The listing builds one solid part. Answer for the finished solid, in the listing's coordinates (mm). A direction names the side the tool comes from. Coordinates: 2 decimals unless noted, no trailing zeros. Loops run counter-clockwise (first coordinate to the right, second up) from the corner with the lowest first, then second, coordinate; pieces in that order, holes last. Notation, with made-up numbers: (48, 79) - (59, 79) arc R18 ccw to (59, 103) - close; hole circle Ø10 at (-12.75, -10.5). An arc over 180 degrees is marked (long way). One line per question, with ' | ' between items.
from build123d import *

# Parameters (mm, degrees)
BOSS_EXTRUDE1_DEPTH      = 6.8
BOSS_EXTRUDE1_DEPTH_BACK = 6.8
CUT_EXTRUDE1_REACH       = 45.967
SKETCH2_R                = 1.1303
SKETCH2_R_2              = 1.7272


with BuildPart() as part:
    # Sketch1 → Boss-Extrude1 (new, two sides: drawn at the far end of the back side and taken through both)
    with BuildSketch(Plane(origin=(0, 0, 0), x_dir=(0, 0, -1), z_dir=(1, 0, 0)).offset(-BOSS_EXTRUDE1_DEPTH_BACK)):
        Polygon((0.889, 3.903), (-0.889, 3.903), (-42.731, 3.903), (-42.731, 2.125), (-0.889, 2.125), (-0.889, -3.903), (3.889, -3.903), (3.889, -2.125), (0.889, -2.125), align=None)
    extrude(amount=BOSS_EXTRUDE1_DEPTH + BOSS_EXTRUDE1_DEPTH_BACK)

    # Sketch2 → Cut-Extrude1 (cut, up to next)
    with BuildSketch(Plane(origin=(0, 3.903, 0), x_dir=(1, 0, 0), z_dir=(0, 1, 0)), mode=Mode.PRIVATE) as cut_extrude1_sk1:
        with Locations(Location((0, -40.8857, 0), (0, 0, 270))):
            Circle(SKETCH2_R)
    cut_extrude1_tool1 = extrude(cut_extrude1_sk1.sketch, amount=-CUT_EXTRUDE1_REACH, mode=Mode.PRIVATE) & part.part
    # Sketch2 → Cut-Extrude1 (cut, up to next)
    with BuildSketch(Plane(origin=(0, 3.903, 0), x_dir=(1, 0, 0), z_dir=(0, 1, 0)), mode=Mode.PRIVATE) as cut_extrude1_sk2:
        with Locations(Location((0, -35.8857, 0), (0, 0, 270))):
            Circle(SKETCH2_R_2)
    cut_extrude1_tool2 = extrude(cut_extrude1_sk2.sketch, amount=-CUT_EXTRUDE1_REACH, mode=Mode.PRIVATE) & part.part
    # Sketch2 → Cut-Extrude1 (cut, up to next)
    with BuildSketch(Plane(origin=(0, 3.903, 0), x_dir=(1, 0, 0), z_dir=(0, 1, 0)), mode=Mode.PRIVATE) as cut_extrude1_sk3:
        with Locations(Location((0, -30.8857, 0), (0, 0, 270))):
            Circle(SKETCH2_R)
    cut_extrude1_tool3 = extrude(cut_extrude1_sk3.sketch, amount=-CUT_EXTRUDE1_REACH, mode=Mode.PRIVATE) & part.part
    add(cut_extrude1_tool1.solids().sort_by_distance((0, 3.903, 40.8857))[0], mode=Mode.SUBTRACT)
    add(cut_extrude1_tool2.solids().sort_by_distance((0, 3.903, 35.8857))[0], mode=Mode.SUBTRACT)
    add(cut_extrude1_tool3.solids().sort_by_distance((0, 3.903, 30.8857))[0], mode=Mode.SUBTRACT)


solid = part.part
Item 1: Each of these flat-tipped pins is pushed along its axis until it touches: pin 1 Ø1 at (y, z) = (0, 2) entering from -X; pin 2 Ø1.5 at (x, y) = (-5, -0.5) entering from +Z; pin 3 Ø2 at (y, z) = (1.5, 29) entering from -X; pin 4 Ø1.5 at (x, z) = (-1, -2) entering from +Y (3 decimals). Where does it stop, or does it pass through?
Taken from the geometry:
pin 1: passes through | pin 2: stops at z = 0.89 | pin 3: stops at x = -6.8 | pin 4: stops at y = -2.125
Item 2: Find the intervals of material crossed by line 1 (Z direction, x = 0, y = 1); line 2 (Z direction, x = -2.75, y = 2.75); line 3 (Y direction, x = 0.75, z = 28) (3 decimals), in increasing order. Write a range as [from, to].
Taken from the geometry:
line 1: z = [-0.89, 0.89] | line 2: z = [-0.89, 42.73] | line 3: y = [2.125, 3.903]
Item 3: Which of the six approach directions +Z, -Z, +X, -X, +Y, -Y give full straight-line access (tool end or side, diameter ignored) to faces 1 (the face through (0, -3, -3.889)), 2 (the face through (0, -1, 0.889)), 3 (the face through (0, 1, -0.889))?
Taken from the geometry:
face 1: -Z, +X, -X, +Y, -Y | face 2: +Z, +X, -X, -Y | face 3: -Z, +X, -X, +Y
Item 4: The mould has two halves that part along Z. Classify faces 4 (the face through (0.34, 3.026, 41.964)), 5 (the face through (0, 3, 42.731)), 6 (the face through (0, -3.903, -1)), 7 (the face through (-0.43, 3.03, 31.93)): pulls with the +Z half, pulls with the -Z half, needs draft (parallel to the pull), parting line crosses it, or undercut.
Taken from the geometry:
face 4: undercut | face 5: pulls with the +Z half | face 6: needs draft | face 7: undercut
Item 5: Find section D-D, the plane z = 27. Write down the section's boundary in (x, y) (3 decimals).
Taken from the geometry:
outline: (-6.8, 2.125) - (6.8, 2.125) - (6.8, 3.903) - (-6.8, 3.903) - close
Item 6: Find section B-B, the plane y = 3.25. Write down the section's boundary in (x, z), plus the area to 3 significant figures.
Taken from the geometry:
outline: (-6.8, -0.89) - (6.8, -0.89) - (6.8, 42.73) - (-6.8, 42.73) - close; hole circle Ø3.45 at (0, 35.89); hole circle Ø2.26 at (0, 30.89); hole circle Ø2.26 at (0, 40.89) | area: 576 mm2
Item 7: Find section A-A, the plane x = 0. Write down the section's boundary in (y, z) (1 decimal).
Taken from the geometry:
outline: (-3.9, -3.9) - (-2.1, -3.9) - (-2.1, -0.9) - (3.9, -0.9) - (3.9, 29.8) - (2.1, 29.8) - (2.1, 0.9) - (-3.9, 0.9) - close; (2.1, 32) - (3.9, 32) - (3.9, 34.2) - (2.1, 34.2) - close; (2.1, 37.6) - (3.9, 37.6) - (3.9, 39.8) - (2.1, 39.8) - close; (2.1, 42) - (3.9, 42) - (3.9, 42.7) - (2.1, 42.7) - close
Item 8: Find section C-C, the plane x = 2.75. Write down the section's boundary in (y, z) (3 decimals), plus the area to 3 significant figures.
Taken from the geometry:
outline: (-3.903, -3.889) - (-2.125, -3.889) - (-2.125, -0.889) - (3.903, -0.889) - (3.903, 42.731) - (2.125, 42.731) - (2.125, 0.889) - (-3.903, 0.889) - close | area: 93.6 mm2
